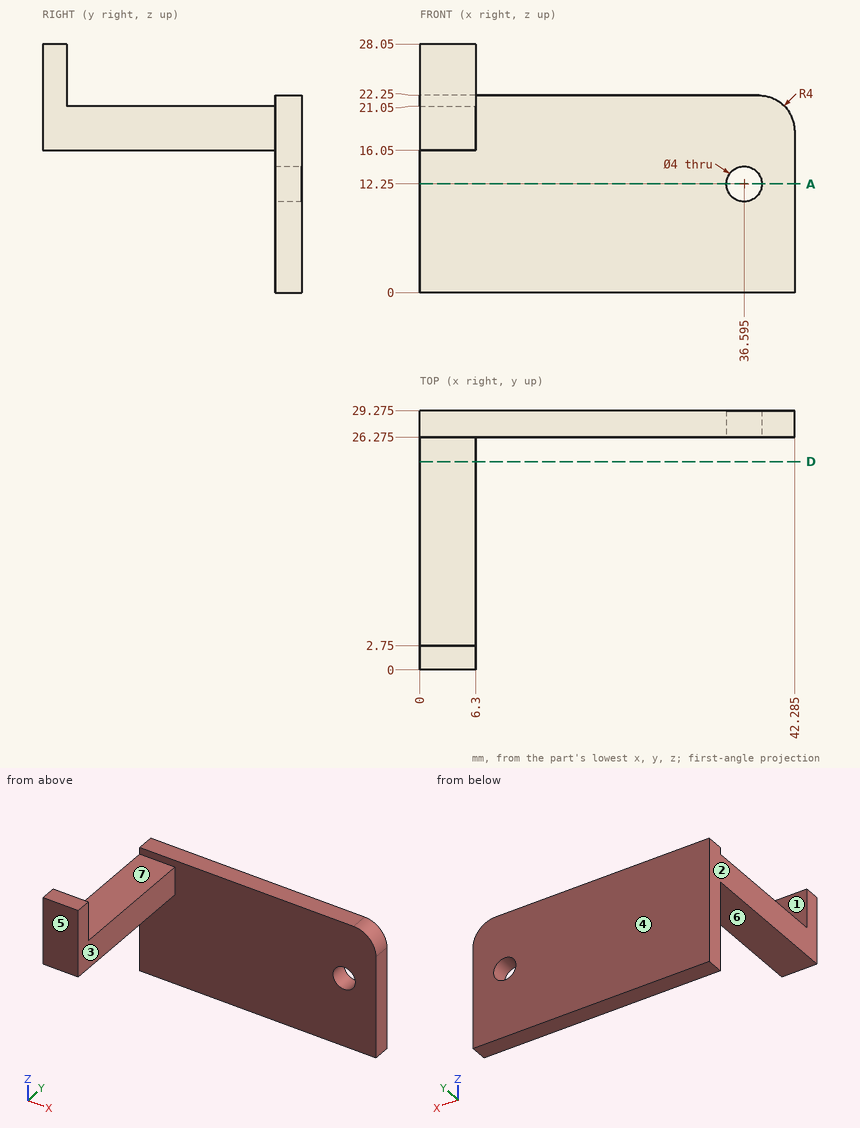
Geometry: see drawing. Coordinates: mm, zero at the bounding-box minimum. A direction names the side the tool comes from. Round coordinates to 2 decimals unless told otherwise and drop trailing zeros. Write each loop counter-clockwise with the first axis right and the second up, starting at its lowest first coordinate (ties: lowest second). Pieces come first, ordered by that corner, then holes.
Item 1: Pin query (flat end, axial travel): P1, Ø5, axis at y = 21.5, z = 19, coming from the +X side; P2, Ø1.9, axis at x = 3.5, y = 10, coming from the +Z side; P3, Ø4, axis at x = 34, z = 20.5, coming from the -Y side (3 decimals). Return the tip coordinate at first contact, or that it passes through.
Item 2: Section query D-D (y = 23.5). Return loops of the section in (x, z).
Item 3: Set-up query: the marked faces 1, 2 and 3. Return all of +Z, -Z, +X, -X, +Y, -Y with unobstructed straight access to the full face (end or side cutting, diameter ignored); none if empty.
Item 4: Mould query, pull axis Y, two halves, no side actions, for the marked faces 4, 5, 6 and 7. Classes: +Y half, -Y half, draft (parallel to the pull), parting line (faces both ways), or undercut.
Item 5: Material intervals for L1, parallel to X at y = 27.3, z = 12.25 (1 decimal); L2, parallel to Y at x = 2, z = 7.25 (1 decimal); L3, parallel to X at y = 11.25, z = 20, sorted ascending.
Item 6: Section query A-A (z = 12.25). Return loops of the section in (x, y) (1 decimal).
Completed:
1. P1: stops at x = 6.3
1. P2: stops at z = 21.05
1. P3: stops at y = 26.275
2. outline: (0, 16.05) - (6.3, 16.05) - (6.3, 21.05) - (0, 21.05) - close
3. face 1: +Z, +X, -X
3. face 2: +Z, -Z, -X, +Y, -Y
3. face 3: +Z, -Z, +X, -Y
4. face 4: +Y half
4. face 5: -Y half
4. face 6: draft
4. face 7: undercut
5. L1: x = 0 to 34.6, 38.6 to 42.3
5. L2: y = 26.3 to 29.3
5. L3: x = 0 to 6.3
6. outline: (0, 26.3) - (34.6, 26.3) - (34.6, 29.3) - (0, 29.3) - close; (38.6, 26.3) - (42.3, 26.3) - (42.3, 29.3) - (38.6, 29.3) - close
